Source: CAD feature listing. Evaluate the final solid. Frame: model axes, mm. Face numbers are marked on the shaded views. A direction names the side the tool comes from. Give positions to 0.01 mm unless a question says otherwise; leave off trailing zeros. Loops run counter-clockwise (first coordinate to the right, second up) from the corner with the lowest first, then second, coordinate; pieces in that order, holes last. Notation, with made-up numbers: M 82,47.5 L 87,47.5 A4 cw 87,52.5 Z; hole C 83,21 d2. An arc over 180 degrees is marked long. Answer in a Markdown table with one row per item.
```python
from build123d import *

# Parameters (mm, degrees)
SKETCH2_W           = 1
SKETCH2_H           = 1
BOSS_EXTRUDE1_DEPTH = 6.5
FILLET1_R           = 1.5


with BuildPart() as part:
    # Sketch2 → Boss-Extrude1 (new body)
    with BuildSketch(Plane.XY):
        with Locations((31.95, 48)):
            Rectangle(SKETCH2_W, SKETCH2_H)
        Polygon((35.75, 56.5), (32.45, 56.5), (32.45, 48.5), (32.45, 47.5), (35.75, 47.5), align=None)
        Polygon((39.05, 56.5), (35.75, 56.5), (35.75, 47.5), (39.05, 47.5), (39.05, 48.5), align=None)
        with Locations((39.55, 48)):
            Rectangle(SKETCH2_W, SKETCH2_H)
    extrude(amount=BOSS_EXTRUDE1_DEPTH)

    # Fillet1
    fillet1_edges = [part.edges().sort_by_distance(p)[0] for p in [
        (32.45, 52.5, 0),
        (35.75, 56.5, 0),
        (39.05, 52.5, 0),
        (32.45, 56.5, 3.25),
        (39.05, 56.5, 3.25),
        (39.05, 52.5, 6.5),
        (35.75, 56.5, 6.5),
        (32.45, 52.5, 6.5),
    ]]
    fillet(fillet1_edges, radius=FILLET1_R)


solid = part.part
```
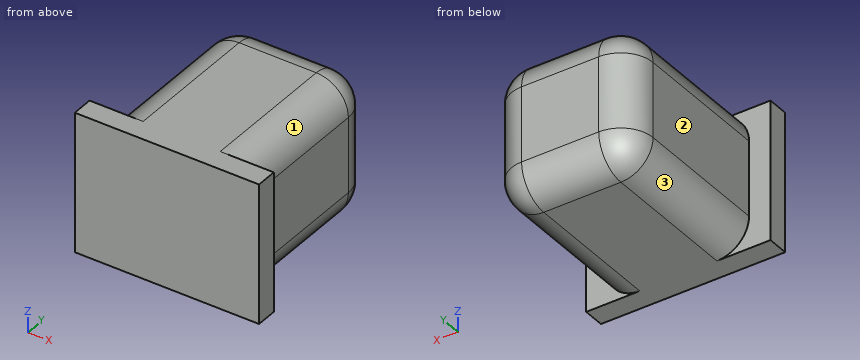
1) Section B-B, the plane z = 3.5. Return loops of the section in (x, y).
Reply:
| item | result |
|---|---|
| outline | M 31.45,47.5 L 40.05,47.5 L 40.05,48.5 L 39.05,48.5 L 39.05,55 A1.5 ccw 37.55,56.5 L 33.95,56.5 A1.5 ccw 32.45,55 L 32.45,48.5 L 31.45,48.5 Z |
2) Material intervals for L1, parallel to X at y = 51.5, z = 2.25; L2, parallel to Y at x = 39.25, z = 0.75; L3, parallel to Z at x = 33, y = 51.5, sorted ascending.
Reply:
| item | result |
|---|---|
| L1 | x = 32.45 to 39.05 |
| L2 | y = 47.5 to 48.5 |
| L3 | z = 0.34 to 6.16 |
3) Set-up query: the marked faces 1, 2 and 3. Return all of +Z, -Z, +X, -X, +Y, -Y with unobstructed straight access to the full face (end or side cutting, diameter ignored); none if empty.
Reply:
| item | result |
|---|---|
| face 1 | +Z, +X, +Y |
| face 2 | +Z, -Z, -X, +Y |
| face 3 | -Z, -X, +Y |
4) Section D-D, the plane z = 0.75. Return loops of the section in (x, y), then the cut area to 3 significant figures.
Reply:
| item | result |
|---|---|
| outline | M 31.45,47.5 L 40.05,47.5 L 40.05,48.5 L 38.85,48.5 L 38.85,55 A1.3 ccw 37.55,56.3 L 33.95,56.3 A1.3 ccw 32.65,55 L 32.65,48.5 L 31.45,48.5 Z |
| area | 56.2 mm² |
5) Pin query (flat end, axial travel): pin 1 Ø1.8 at (y, z) = (52, 3) entering from -X; pin 2 Ø1.8 at (y, z) = (51.5, 3) entering from +X; pin 3 Ø1 at (x, y) = (39, 54.5) entering from +Z. Return the tip coordinate at first contact, or that it passes through.
Reply:
| item | result |
|---|---|
| pin 1 | stops at x = 32.45 |
| pin 2 | stops at x = 39.05 |
| pin 3 | stops at z = 6.16 |
6) Section C-C, the plane x = 37. Return loops of the section in (y, z).
Reply:
| item | result |
|---|---|
| outline | M 47.5,0 L 55,0 A1.5 ccw 56.5,1.5 L 56.5,5 A1.5 ccw 55,6.5 L 47.5,6.5 Z |
7) Section A-A, the plane y = 50.75. Return loops of the section in (x, z), then the cut area to 3 significant figures.
Reply:
| item | result |
|---|---|
| outline | M 32.45,1.5 A1.5 ccw 33.95,0 L 37.55,0 A1.5 ccw 39.05,1.5 L 39.05,5 A1.5 ccw 37.55,6.5 L 33.95,6.5 A1.5 ccw 32.45,5 Z |
| area | 41.0 mm² |
